Model file for the job. Use its own axes, mm. Face numbers are marked on the shaded views. Coordinates: 2 decimals unless noted, no trailing zeros. Loops run counter-clockwise (first coordinate to the right, second up) from the corner with the lowest first, then second, coordinate; pieces in that order, holes last. Notation, with made-up numbers: M 58,-27.75 L 73,-27.75 A18 ccw 73,1.25 Z; hole C 49,59 d2. An arc over 180 degrees is marked long. Write item = value, one per line. Start each with the question number.
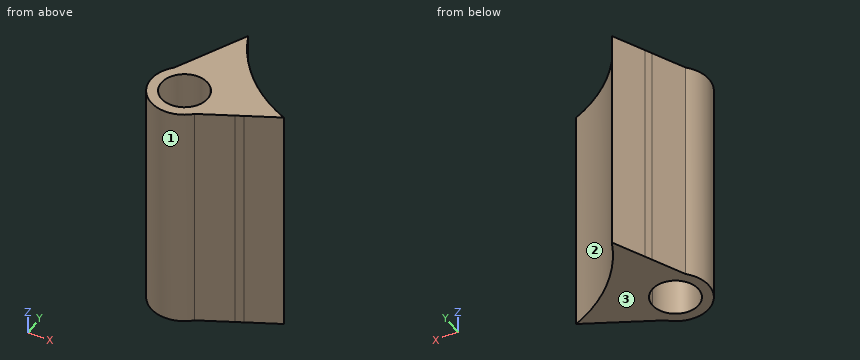
from build123d import *

# Parameters (mm, degrees)
F1_DEPTH = 25.4


with BuildPart() as f1:
    # F0 (on Top) → F1 (new body)
    with BuildSketch(Plane.XY):
        with BuildLine():
            Line((-0.898026, 6.106574), (-2.604274, 2.604274))
            ThreePointArc((-2.604274, 2.604274), (-2.604274, -2.604274), (2.604274, -2.604274))
            Line((2.604274, -2.604274), (6.106574, -0.898026))
            Line((6.106574, -0.898026), (6.867985, -0.527082))
            Line((6.867985, -0.527082), (10.309378, 1.149494))
            ThreePointArc((10.309378, 1.149494), (4.849338, 4.849338), (1.149494, 10.309378))
            Line((1.149494, 10.309378), (-0.527082, 6.867985))
            Line((-0.527082, 6.867985), (-0.898026, 6.106574))
        make_face()
        with BuildLine():
            ThreePointArc((1.796051, 1.796051), (2.346654, 0.972016), (2.54, 0))
            ThreePointArc((2.54, 0), (-2.346654, -0.972016), (1.796051, 1.796051))
        make_face(mode=Mode.SUBTRACT)
    extrude(amount=F1_DEPTH)


solid = f1.part
Item 1: Cut at C-C (x = 0). Give the cut face in (y, z), plus the area to 3 significant figures.
Item 2: Cut at B-B (x = -1.5). Give the cut face in (y, z), plus the area to 3 significant figures.
Item 3: Pull direction X, two halves, no side cores. Call the marked faces 1, 2 and 3: +X half, -X half, draft (parallel to the pull), parting line (faces both ways), or undercut.
Item 4: Cut at D-D (y = 4.5). Give the cut face in (x, z), plus the area to 3 significant figures.
Item 5: Probe L1, parallel to X at y = 1.5, z = 15.5; L2, parallel to Y at x = 0, z = 11; L3, parallel to X at y = 0.25, z = 12. List the from-to ranges inside material, lowest first.
Item 6: Pin check, flat tips, straight feed: pin 1 Ø4 at (y, z) = (2, 13.5) entering from +X; pin 2 Ø5 at (x, z) = (4.5, 16) entering from -Y; pin 3 Ø5 at (x, z) = (9, 6.5) entering from -Y. Stop position of each tip, or through.
Reported:
q1.outline = M -3.68,0 L -2.54,0 L -2.54,25.4 L -3.68,25.4 Z; M 2.54,0 L 7.95,0 L 7.95,25.4 L 2.54,25.4 Z
q1.area = 166 mm^2
q2.outline = M -3.36,0 L -2.05,0 L -2.05,25.4 L -3.36,25.4 Z; M 2.05,0 L 4.87,0 L 4.87,25.4 L 2.05,25.4 Z
q2.area = 105 mm^2
q3.face_1 = parting line
q3.face_2 = +X half
q3.face_3 = draft
q4.outline = M -1.68,0 L 5.21,0 L 5.21,25.4 L -1.68,25.4 Z
q4.area = 175 mm^2
q5.L1 = -3.36 to -2.05, 2.05 to 9.54
q5.L2 = -3.68 to -2.54, 2.54 to 7.95
q5.L3 = -3.67 to -2.53, 2.53 to 8.46
q6.pin_1 = 10.31
q6.pin_2 = -3.09
q6.pin_3 = -0.71
